For this review, use the dimensioned drawing (mm, ordinates from the lowest corner) and the shaded views. A direction names the side the tool comes from. Coordinates: 2 decimals unless noted, no trailing zeros. Write each loop counter-clockwise with the first axis right and the second up, starting at its lowest first coordinate (ties: lowest second). Pieces come first, ordered by that corner, then holes. Notation, with made-up numbers: (86.5, 44.25) - (96.5, 44.25) arc R13 cw to (96.5, 63.25) - close; hole circle Ø3 at (34, 42). An arc over 180 degrees is marked (long way). Use one line per item in the form item = value. Start each with the question number.
1) We need section D-D (x = 115). Give the boundary of the cut face in (y, z).
2) Insertion check: P1, Ø2, axis at x = 188, z = 97.5, coming from the -Y side; P2, Ø4, axis at x = 225, y = 20, coming from the -Z side; P3, Ø10, axis at x = 74, z = 87.5, coming from the +Y side. Each pin has a flat end and moves straight along its axis. Give the tip position at first contact, or say it passes through.
3) We need section C-C (x = 190). Give the boundary of the cut face in (y, z), plus the area to 3 significant figures.
4) For L1, parallel to Z at x = 145.5, y = 17; L2, parallel to Y at x = 225, z = 7; L3, parallel to X at y = 2, z = 76, list the stretches that pass through material, from the lowest coordinate up. Write a range as from..to.
5) We need section B-B (x = 226). Give the boundary of the cut face in (y, z).
6) We need section A-A (z = 65). Give the boundary of the cut face in (x, y).
7) Mouldability with a two-part tool opening along Z and no side actions: class the marked faces 4, 5 and 6 as pulls with the +Z half, pulls with the -Z half, needs draft (parallel to the pull), parting line crosses it, or undercut.
8) Tool access review of the marked faces 1, 2 and 3: name each direction out of +Z, -Z, +X, -X, +Y, -Y from which nothing blocks a thin tool from reaching the whole face with its end or side.
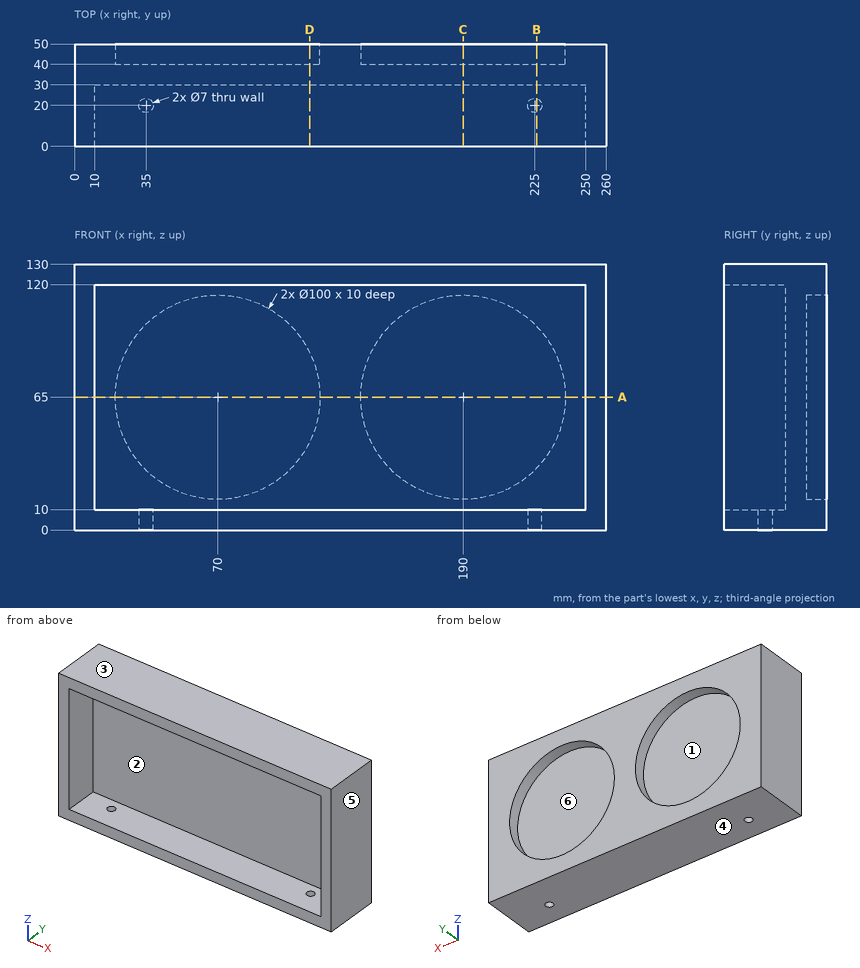
Determined:
q1.outline = (0, 0) - (50, 0) - (50, 43.21) - (40, 43.21) - (40, 86.79) - (50, 86.79) - (50, 130) - (0, 130) - (0, 120) - (30, 120) - (30, 10) - (0, 10) - close
q2.P1 = 30
q2.P2 = 120
q2.P3 = 40
q3.outline = (0, 0) - (50, 0) - (50, 15) - (40, 15) - (40, 115) - (50, 115) - (50, 130) - (0, 130) - (0, 120) - (30, 120) - (30, 10) - (0, 10) - close
q3.area = 2,200 mm²
q4.L1 = 0..10, 120..130
q4.L2 = 0..16.5, 23.5..50
q4.L3 = 0..10, 250..260
q5.outline = (0, 0) - (16.65, 0) - (16.65, 10) - (0, 10) - close; (0, 120) - (30, 120) - (30, 10) - (23.35, 10) - (23.35, 0) - (50, 0) - (50, 30.3) - (40, 30.3) - (40, 99.7) - (50, 99.7) - (50, 130) - (0, 130) - close
q6.outline = (0, 0) - (10, 0) - (10, 30) - (250, 30) - (250, 0) - (260, 0) - (260, 50) - (240, 50) - (240, 40) - (140, 40) - (140, 50) - (120, 50) - (120, 40) - (20, 40) - (20, 50) - (0, 50) - close
q7.face_4 = pulls with the -Z half
q7.face_5 = needs draft
q7.face_6 = undercut
q8.face_1 = +Y
q8.face_2 = -Y
q8.face_3 = +Z, +X, -X, +Y, -Y
